The drawing under review shows one solid part. Ordinate dimensions are in mm from its lowest x, y, z. A direction names the side the tool comes from. Round coordinates to 2 decimals unless told otherwise and drop trailing zeros. Write each loop counter-clockwise with the first axis right and the second up, starting at its lowest first coordinate (ties: lowest second). Pieces come first, ordered by that corner, then holes. Notation, with made-up numbers: (66.25, 18) -> (70.25, 18) arc R15 cw to (70.25, 29) -> close; hole circle Ø1 at (3, -39). An arc over 180 degrees is marked (long way). Answer in a Markdown table with one row per item.
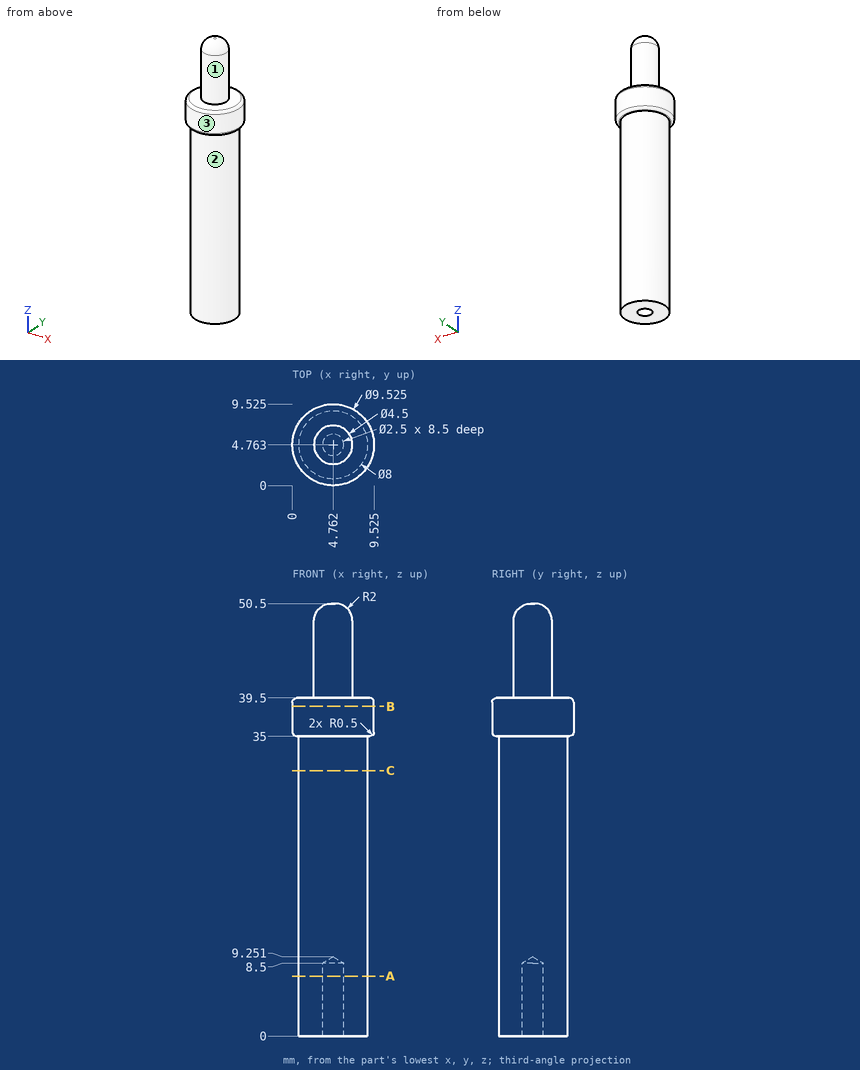
1) Consider section C-C on z = 31. State the section outline as (x, y) points.
Solved:
| item | result |
|---|---|
| outline | circle Ø8 at (4.76, 4.76) |
2) Consider section A-A on z = 7. State the section outline as (x, y) points.
Solved:
| item | result |
|---|---|
| outline | circle Ø8 at (4.76, 4.76); hole circle Ø2.5 at (4.76, 4.76) |
3) Clearance check with flat-ended pins moving along their axes: pin 1 Ø5 at (x, z) = (7, 30) entering from -Y; pin 2 Ø5 at (y, z) = (2, 5.5) entering from +X; pin 3 Ø1.5 at (x, z) = (1.5, 5.5) entering from -Y. State where each tip first meets the part, or that it passes through.
Solved:
| item | result |
|---|---|
| pin 1 | y = 0.76 |
| pin 2 | x = 8.75 |
| pin 3 | y = 1.65 |
4) For line 1 (Y direction, x = 4.75, z = 7.5); line 2 (Z direction, x = 2, y = 6.75); line 3 (X direction, y = 4.5, z = 19) (1 decimal), list the stretches that pass through material, from the lowest coordinate up. Write a range as [from, to].
Solved:
| item | result |
|---|---|
| line 1 | [0.76, 3.51], [6.01, 8.76] |
| line 2 | [0, 39.5] |
| line 3 | [0.8, 8.8] |
5) Consider section B-B on z = 38.5. State the section outline as (x, y) points (1 decimal).
Solved:
| item | result |
|---|---|
| outline | circle Ø9.5 at (4.8, 4.8) |
6) For the marked faces 1, 2 and 3, list the 3-axis set-ups (+Z, -Z, +X, -X, +Y, -Y) from which the entire face can be reached by the end or side of a thin tool; tool diameter is ignored.
Solved:
| item | result |
|---|---|
| face 1 | +Z |
| face 2 | -Z |
| face 3 | +Z, -Z |
